Can you work these out from the model? Positions are in its coordinate system, mm. A direction names the side the tool comes from. Give positions to 0.01 mm unless a question says otherwise; leave off trailing zeros. Order: outer loops, then holes, each group sorted by start corner. A loop starts at its lowest first (then second) coordinate and runs counter-clockwise, first axis right, second up. Notation, with made-up numbers: (-1.5, 53.5) - (24.5, 53.5) arc R7 ccw to (24.5, 61.5) - close; hole circle Ø1 at (-22.5, 69). An arc over 180 degrees is marked (long way). Return JSON: item names as keys, results as strings.
```python
from build123d import *

# Parameters (mm, degrees)
F1_DEPTH      = 30
F1_DEPTH_BACK = 30
F2_R          = 19
F2_R_2        = 3
F3_DEPTH      = 6.001
F5_DEPTH      = 25


with BuildPart() as f1:
    # F0 (on Front) → F1 (new body, two sides)
    with BuildSketch(Plane.XZ) as f1_sk:
        Polygon((0, 70), (0, 0), (70, 0), (70, 6), (6, 6), (6, 70), align=None)
    extrude(amount=F1_DEPTH)
    extrude(f1_sk.sketch, amount=-F1_DEPTH_BACK)

    # F2 (on face) → F3 (cut, through all)
    with BuildSketch(Plane.YZ.offset(6)):
        with Locations((0, 40)):
            Circle(F2_R)
        with Locations((-23.5, 63.5)):
            Circle(F2_R_2)
        with Locations((-23.5, 16.5)):
            Circle(F2_R_2)
        with Locations((23.5, 16.5)):
            Circle(F2_R_2)
        with Locations((23.5, 63.5)):
            Circle(F2_R_2)
    extrude(amount=-F3_DEPTH, mode=Mode.SUBTRACT)

    # F4 (on face) → F5 (cut)
    with BuildSketch(Plane.XY.offset(6)):
        with BuildLine():
            ThreePointArc((29, -18.5), (32.5, -15), (29, -11.5))
            Line((29, -11.5), (17, -11.5))
            ThreePointArc((17, -11.5), (13.5, -15), (17, -18.5))
            Line((17, -18.5), (29, -18.5))
        make_face()
        with BuildLine():
            ThreePointArc((59, -18.5), (62.5, -15), (59, -11.5))
            Line((59, -11.5), (47, -11.5))
            ThreePointArc((47, -11.5), (43.5, -15), (47, -18.5))
            Line((47, -18.5), (59, -18.5))
        make_face()
        with BuildLine():
            Line((47, 11.5), (59, 11.5))
            ThreePointArc((59, 11.5), (62.5, 15), (59, 18.5))
            Line((59, 18.5), (47, 18.5))
            ThreePointArc((47, 18.5), (43.5, 15), (47, 11.5))
        make_face()
        with BuildLine():
            ThreePointArc((29, 11.5), (32.5, 15), (29, 18.5))
            Line((29, 18.5), (17, 18.5))
            ThreePointArc((17, 18.5), (13.5, 15), (17, 11.5))
            Line((17, 11.5), (29, 11.5))
        make_face()
    extrude(amount=-F5_DEPTH, mode=Mode.SUBTRACT)


solid = f1.part
```
1. For pin 1 Ø5 at (y, z) = (23.5, 16.5) entering from +X; pin 2 Ø12 at (y, z) = (-23.5, 18) entering from +X; pin 3 Ø8 at (x, y) = (19, -13.5) entering from -Z, each with a flat end and sliding along its axis, tell me the tip position at first contact or that it passes through.
Checks:
{"pin 1": "through", "pin 2": "x = 6", "pin 3": "z = 0"}
2. If I drill on L1, parallel to Z at x = 3.25, y = 23.5; L2, parallel to Z at x = 62.5, y = 10; L3, parallel to Z at x = 3.7, y = 0, over which ranges is the centre line in solid material (lowest first)? Write a range as [from, to].
Checks:
{"L1": "[0, 13.5], [19.5, 60.5], [66.5, 70]", "L2": "[0, 6]", "L3": "[0, 21], [59, 70]"}
3. Thinking about a two-plate mould opening in X: for faces 3 (the face through (4, 30, 20)), 4 (the face through (6, -14, 23)), 5 (the face through (53, 11.5, 3)), which applies, +X half, -X half, draft (parallel to the pull), parting line (faces both ways), or undercut?
Checks:
{"face 3": "draft", "face 4": "+X half", "face 5": "undercut"}
4. Suppose I cut it at B-B (x = 26). List the corners of the cut face in (y, z) for me.
Checks:
{"outline": "(-30, 0) - (-18.5, 0) - (-18.5, 6) - (-30, 6) - close; (-11.5, 0) - (11.5, 0) - (11.5, 6) - (-11.5, 6) - close; (18.5, 0) - (30, 0) - (30, 6) - (18.5, 6) - close"}
5. Suppose I cut it at A-A (z = 40). List the corners of the cut face in (x, y) for me.
Checks:
{"outline": "(0, -30) - (6, -30) - (6, -19) - (0, -19) - close; (0, 19) - (6, 19) - (6, 30) - (0, 30) - close"}
6. Suppose I cut it at C-C (y = -23.5). List the corners of the cut face in (x, z) for me.
Checks:
{"outline": "(0, 0) - (70, 0) - (70, 6) - (6, 6) - (6, 13.5) - (0, 13.5) - close; (0, 19.5) - (6, 19.5) - (6, 60.5) - (0, 60.5) - close; (0, 66.5) - (6, 66.5) - (6, 70) - (0, 70) - close"}
7. On a 3-axis mill with a long thin cutter (end or side, diameter ignored), from which of +Z, -Z, +X, -X, +Y, -Y can I reach the whole of each face in a straight line? I mean faces 1 (the face through (4, -30, 20)), 2 (the face through (23, 18.5, 3)). Say none if no direction works.
Checks:
{"face 1": "+Z, -Z, +X, -X, -Y", "face 2": "+Z, -Z"}
8. Suppose I cut it at D-D (z = 63.5). List the corners of the cut face in (x, y) for me, plus the area to 3 significant figures.
Checks:
{"outline": "(0, -30) - (6, -30) - (6, -26.5) - (0, -26.5) - close; (0, -20.5) - (6, -20.5) - (6, 20.5) - (0, 20.5) - close; (0, 26.5) - (6, 26.5) - (6, 30) - (0, 30) - close", "area": "288 mm^2"}
